```python
from build123d import *

# Parameters (mm, degrees)
F0_W        = 18
F0_H        = 8
F0_R        = 1.5
F1_DEPTH    = 4
F0_W_2      = 12
F0_H_2      = 2.5
F2_DEPTH    = 31.5
F3_R        = 3.5
F4_DEPTH    = 12.001
F5_R        = 5
F6_DEPTH    = 2
F8_SIZE     = 2.4
F9_T1_DEPTH = 143.1852716253


# Not quite as in the source:
# - a fillet or chamfer that OpenCascade refuses, or shapes differently, is made with other operations: its cross-section is extruded or revolved along the edge and cut away or added


with BuildPart() as f1:
    # F0 (on Top) → F1 (new body)
    with BuildSketch(Plane.XY):
        with Locations((6, 0)):
            Rectangle(F0_W, F0_H)
        with Locations((2, 0)):
            Circle(F0_R, mode=Mode.SUBTRACT)
        with Locations((10, 0)):
            Circle(F0_R, mode=Mode.SUBTRACT)
    extrude(amount=F1_DEPTH)

    # F0 (on Top) → F2 (join)
    with BuildSketch(Plane.XY):
        with Locations((-9, -5.25)):
            Rectangle(F0_W_2, F0_H_2)
        with Locations((-9, 0)):
            Rectangle(F0_W_2, F0_H)
        with Locations((-9, 5.25)):
            Rectangle(F0_W_2, F0_H_2)
    extrude(amount=F2_DEPTH)

    # F3 (on face) → F4 (cut, through all)
    with BuildSketch(Plane.YZ.offset(-3)):
        Polygon((-6.5, 0), (-4, 0), (-6.5, 25), align=None)
        Polygon((6.5, 25), (4, 0), (6.5, 0), align=None)
        with Locations((0, 25)):
            Circle(F3_R)
    extrude(amount=-F4_DEPTH, mode=Mode.SUBTRACT)

    # F5
    f5_edges = [f1.edges().sort_by_distance(p)[0] for p in [
        (-9, 6.5, 31.5),
        (-9, -6.5, 31.5),
    ]]
    fillet(f5_edges, radius=F5_R)

    # F0 (on Top) → F6 (join)
    with BuildSketch(Plane.XY):
        with Locations((6, 0)):
            Rectangle(F0_W, F0_H)
        with Locations((2, 0)):
            Circle(F0_R, mode=Mode.SUBTRACT)
        with Locations((10, 0)):
            Circle(F0_R, mode=Mode.SUBTRACT)
        with Locations((-9, 0)):
            Rectangle(F0_W_2, F0_H)
    extrude(amount=-F6_DEPTH)

    # F7: chamfer of 2 on 1 edges, made by hand

    # F7_s1 → F7_t2 (revolve, cut)
    with BuildSketch(Plane.XZ):
        Polygon((3.5, 0), (5.5, -2), (3.5, -2), align=None)
    revolve(axis=Axis((2, 0, -2), (0, 0, 1)), mode=Mode.SUBTRACT)

    # F8
    f8_edges = [f1.edges().sort_by_distance(p)[0] for p in [
        (8.5, 0, -2),
    ]]
    chamfer(f8_edges, length=F8_SIZE)

    # F9: chamfer of 2 x 26 on 1 edges, made by hand

    # F9_s2 → F9_t1 (cut)
    with BuildSketch(Plane.XZ.offset(-71.5926358126)):
        Polygon((-11, -2), (15, 0), (15, -2), align=None)
    extrude(amount=F9_T1_DEPTH, mode=Mode.SUBTRACT)


solid = f1.part
```
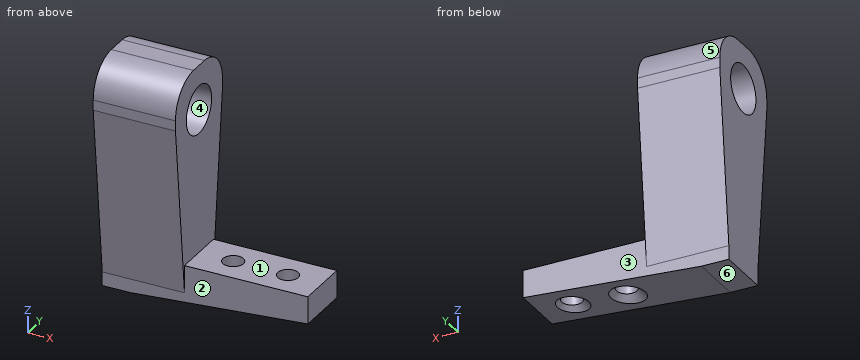
Build history of the part. All positions in model axes, mm. Face numbers are marked on the shaded views. A direction names the side the tool comes from. Give positions to 0.01 mm unless a question says otherwise; leave off trailing zeros. Order: outer loops, then holes, each group sorted by start corner. A loop starts at its lowest first (then second) coordinate and runs counter-clockwise, first axis right, second up. Notation, with made-up numbers: M 71.25,85 L 77.25,85 A28 cw 77.25,121 Z; hole C 66.25,-39 d2. An arc over 180 degrees is marked long. Write item = value, one per line. Start each with the question number.
(1) Slice it at C-C on z = 26. Write the cut outline in (x, y).
(2) Slice it at B-B on x = 2. Write the cut outline in (y, z), plus the area to 3 significant figures.
(3) Pin check, flat tips, straight feed: pin 1 Ø10 at (x, z) = (-4.5, 23.5) entering from +Y; pin 2 Ø6.5 at (y, z) = (1.5, 15) entering from +X; pin 3 Ø5 at (x, z) = (-2.5, 2.5) entering from -Y; pin 4 Ø3 at (x, z) = (2, 0) entering from +Y. Stop position of each tip, or through.
(4) Two-plate mould, pull along Y, no slides. Class the marked faces 4, 5 and 6: released by +Y, released by -Y, zero draft, split by the parting line, or undercut.
(5) Probe L1, parallel to X at y = -0.75, z = 1; L2, parallel to X at y = -3.25, z = 27.5; L3, parallel to Z at x = -5, y = 2.75. List the from-to ranges inside material, lowest first. Write a range as [from, to].
(6) Slice it at A-A on z = 2. Write the cut outline in (x, y).
(7) Slice it at D-D on z = 17. Write the cut outline in (x, y).
(8) Which spindle directions (+Z, -Z, +X, -X, +Y, -Y) get a long thin tool onto all of the face, cutting with end or side? Do the marked faces 1, 2 and 3. Say none if no direction does.
Responses:
q1.outline = M -15,-6.5 L -3,-6.5 L -3,-3.35 L -15,-3.35 Z; M -15,3.35 L -3,3.35 L -3,6.5 L -15,6.5 Z
q2.outline = M -4,-1 L -2.5,-1 L -1.5,0 L -1.5,4 L -4,4 Z; M 1.5,0 L 2.5,-1 L 4,-1 L 4,4 L 1.5,4 Z
q2.area = 24.0 mm2
q3.pin_1 = 6.5
q3.pin_2 = -3
q3.pin_3 = -4.49
q3.pin_4 = 4
q4.face_4 = undercut
q4.face_5 = released by +Y
q4.face_6 = zero draft
q5.L1 = [-15, 0.7], [3.3, 8.7], [11.3, 15]
q5.L2 = [-15, -3]
q5.L3 = [-1.54, 22.83], [27.17, 31.34]
q6.outline = M -15,-4.2 L -3,-4.2 L -3,-4 L 15,-4 L 15,4 L -3,4 L -3,4.2 L -15,4.2 Z; hole C 2,0 d3; hole C 10,0 d3
q7.outline = M -15,-5.7 L -3,-5.7 L -3,5.7 L -15,5.7 Z
q8.face_1 = +Z, +X, +Y, -Y
q8.face_2 = -Z, +X, -Y
q8.face_3 = -Z, +X, +Y
